```python
from build123d import *

# Parameters (mm, degrees)
F0_W     = 6.35
F0_H     = 12.7
F1_DEPTH = 1.5875
F2_W     = 93.517256
F2_H     = 11.267142
F2_R     = 3.175
F3_DEPTH = 1.5875
F4_R     = 3.175
F4_R_2   = 2.54
F5_DEPTH = 1.5875


with BuildPart() as f1:
    # F0 (on Top) → F1 (new body)
    with BuildSketch(Plane.XY):
        with BuildLine():
            Line((0, 12.7), (0, 0))
            Line((0, 0), (127, 0))
            Line((127, 0), (127, 12.7))
            Line((127, 12.7), (127, 34.925))
            Line((127, 34.925), (104.775, 34.925))
            ThreePointArc((104.775, 34.925), (101.6, 31.75), (98.425, 34.925))
            Line((98.425, 34.925), (79.375, 34.925))
            ThreePointArc((79.375, 34.925), (76.2, 31.75), (73.025, 34.925))
            Line((73.025, 34.925), (53.975, 34.925))
            ThreePointArc((53.975, 34.925), (50.8, 31.75), (47.625, 34.925))
            Line((47.625, 34.925), (28.575, 34.925))
            ThreePointArc((28.575, 34.925), (25.4, 31.75), (22.225, 34.925))
            Line((22.225, 34.925), (0, 34.925))
            Line((0, 34.925), (0, 12.7))
        make_face()
        with Locations((-3.175, 6.35)):
            Rectangle(F0_W, F0_H)
        with Locations((-3.175, 47.625)):
            Rectangle(F0_W, F0_H)
        with BuildLine():
            Line((0, 41.275), (0, 34.925))
            Line((0, 34.925), (22.225, 34.925))
            ThreePointArc((22.225, 34.925), (25.4, 38.1), (28.575, 34.925))
            Line((28.575, 34.925), (47.625, 34.925))
            ThreePointArc((47.625, 34.925), (50.8, 38.1), (53.975, 34.925))
            Line((53.975, 34.925), (73.025, 34.925))
            ThreePointArc((73.025, 34.925), (76.2, 38.1), (79.375, 34.925))
            Line((79.375, 34.925), (98.425, 34.925))
            ThreePointArc((98.425, 34.925), (101.6, 38.1), (104.775, 34.925))
            Line((104.775, 34.925), (127, 34.925))
            Line((127, 34.925), (127, 41.275))
            Line((127, 41.275), (127, 53.975))
            Line((127, 53.975), (0, 53.975))
            Line((0, 53.975), (0, 41.275))
        make_face()
        Polygon((127, 34.925), (127, 12.7), (133.35, 12.7), (133.35, 41.275), (127, 41.275), align=None)
    extrude(amount=F1_DEPTH)

    # F2 (on face) → F3 (join)
    with BuildSketch(Plane(origin=(0, 0, 0), x_dir=(1, 0, 0), z_dir=(0, 0, -1))):
        with Locations((62.18549, -34.874498)):
            Rectangle(F2_W, F2_H)
        with Locations((25.4, -34.925)):
            Circle(F2_R, mode=Mode.SUBTRACT)
        with Locations((50.8, -34.925)):
            Circle(F2_R, mode=Mode.SUBTRACT)
        with Locations((76.2, -34.925)):
            Circle(F2_R, mode=Mode.SUBTRACT)
        with Locations((101.6, -34.925)):
            Circle(F2_R, mode=Mode.SUBTRACT)
    extrude(amount=F3_DEPTH)

    # F4 (on face) → F5 (join)
    with BuildSketch(Plane(origin=(0, 0, -1.5875), x_dir=(1, 0, 0), z_dir=(0, 0, -1))):
        with Locations((101.6, -34.925)):
            Circle(F4_R)
        with Locations((101.6, -34.925)):
            Circle(F4_R_2, mode=Mode.SUBTRACT)
        with Locations((76.2, -34.925)):
            Circle(F4_R)
        with Locations((76.2, -34.925)):
            Circle(F4_R_2, mode=Mode.SUBTRACT)
        with Locations((50.8, -34.925)):
            Circle(F4_R)
        with Locations((50.8, -34.925)):
            Circle(F4_R_2, mode=Mode.SUBTRACT)
        with Locations((25.4, -34.925)):
            Circle(F4_R)
        with Locations((25.4, -34.925)):
            Circle(F4_R_2, mode=Mode.SUBTRACT)
    extrude(amount=-F5_DEPTH)


solid = f1.part
```
Geometry check sheet. Reference: the model listing, model coordinates, mm. A direction names the side the tool comes from. Give positions to 0.01 mm unless a question says otherwise; leave off trailing zeros. Loops run counter-clockwise (first coordinate to the right, second up) from the corner with the lowest first, then second, coordinate; pieces in that order, holes last. Notation, with made-up numbers: M 16.5,-8.5 L 70.5,-8.5 A15 ccw 70.5,18.5 Z; hole C 27.25,39 d10. An arc over 180 degrees is marked long. Write item = value, one per line. Start each with the question number.
1. Section check B-B, the plane z = -0.6. Enter the section's corners in (x, y) (3 decimals), plus the area to 3 significant figures.
2. Go/stop test with flat-tipped pins: P1, Ø0.5, axis at x = 72, z = -1, coming from the -Y side; P2, Ø1.3, axis at x = 129, z = 0.5, coming from the +Y side (3 decimals); P3, Ø1.3, axis at y = 37.5, z = -1, coming from the +X side. Record where each tip stops, or that it passes through.
3. Section check C-C, the plane x = 30.5. Enter the section's corners in (y, z) (1 decimal).
4. Section check D-D, the plane y = 8.5. Enter the section's corners in (x, z).
5. Draft check along X on faces 1 (the face through (48, 36, 0)), 2 (the face through (62, 35, -1.588)). Enter one of: +X half, -X half, draft (parallel to the pull), parting line (faces both ways), or undercut.
6. Thickness scan on probe 1 along Y at (x, z) = (76.2, 0.45) (3 decimals); probe 2 along Y at (x, z) = (-0.5, 1.05) (3 decimals); probe 3 along Z at (x, y) = (4, 36). Record the ranges inside material, lowest first.
7. Tool access check on faces 3 (the face through (63, 27, 1.588)), 4 (the face through (23.69, 37.6, 0.78)). Record the directions out of +Z, -Z, +X, -X, +Y, -Y that give a thin tool (end or side, any length) a straight path to the whole face; none if there is none.
Values follow:
q1.outline = M 15.427,29.241 L 108.944,29.241 L 108.944,40.508 L 15.427,40.508 Z; hole C 25.4,34.925 d5.08; hole C 50.8,34.925 d5.08; hole C 76.2,34.925 d5.08; hole C 101.6,34.925 d5.08
q1.area = 973 mm^2
q2.P1 = 29.24
q2.P2 = 41.275
q2.P3 = 108.94
q3.outline = M 0,0 L 29.2,0 L 29.2,-1.6 L 40.5,-1.6 L 40.5,0 L 54,0 L 54,1.6 L 0,1.6 Z
q4.outline = M -6.35,0 L 127,0 L 127,1.59 L -6.35,1.59 Z
q5.face_1 = undercut
q5.face_2 = draft
q6.probe_1 = 0 to 31.75, 38.1 to 53.975
q6.probe_2 = 0 to 12.7, 41.275 to 53.975
q6.probe_3 = 0 to 1.59
q7.face_3 = +Z, +X, -X, +Y, -Y
q7.face_4 = +Z
